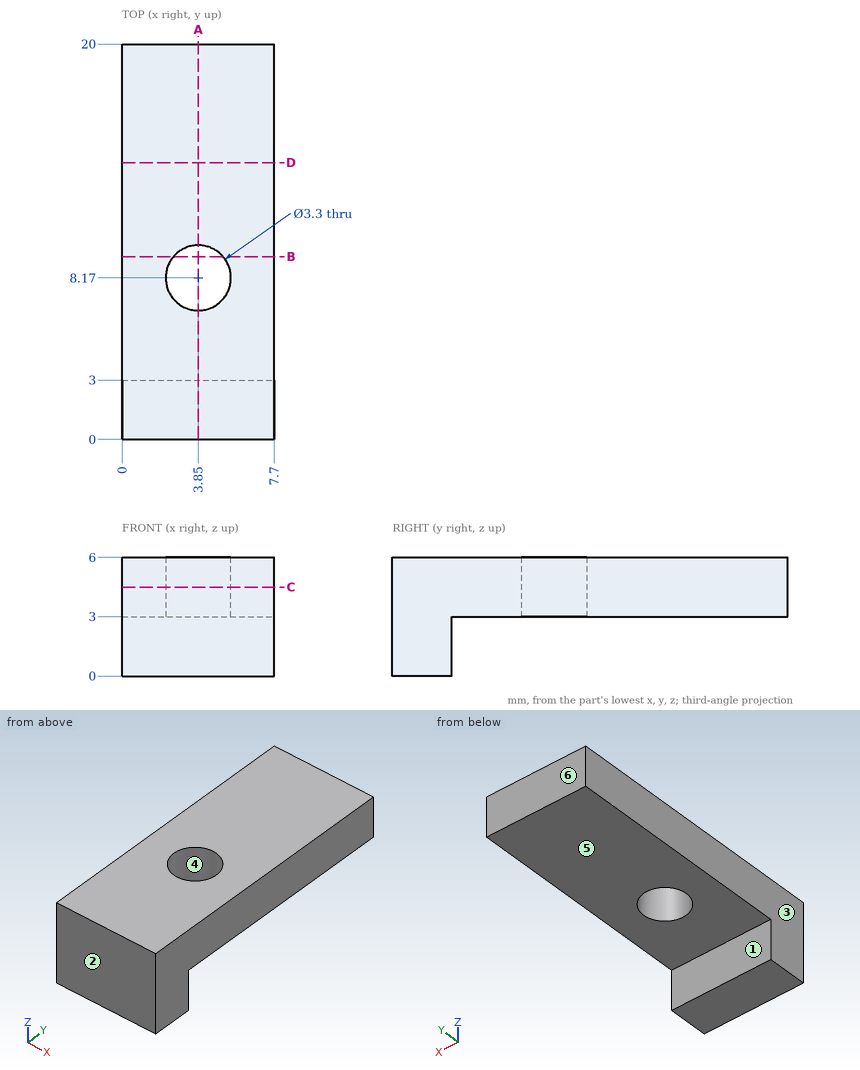
Study the drawing (mm; zero at the part's minimum x, y, z) and answer. A direction names the side the tool comes from. Coordinates: 2 decimals unless noted, no trailing zeros. Loops run counter-clockwise (first coordinate to the right, second up) from the corner with the lowest first, then second, coordinate; pieces in that order, holes last. Notation, with made-up numbers: M 56,83 L 111,83 A21 ccw 111,117 Z; hole C -32,-8.75 d2. An arc over 180 degrees is marked long. Answer in a Markdown table with one row per item. Add a question column.
1. Consider L1, parallel to Y at x = 3.85, z = 3.75; L2, parallel to Z at x = 0.5, y = 17.25; L3, parallel to Y at x = 1.5, z = 2.8. Determine where each line is inside the solid, lowest interval first.
2. The mould has two halves that part along Y. Classify the marked faces 1, 2, 3 and 4: pulls with the +Y half, pulls with the -Y half, needs draft (parallel to the pull), parting line crosses it, or undercut.
3. Find section B-B, the plane y = 9.25. Write down the section's boundary in (x, z).
4. A tool of negligible diameter and unlimited length cuts with its end or side. For the marked faces 5 and 6, from which of +Z, -Z, +X, -X, +Y, -Y can it reach the whole face along a straight path? Write none if from no direction.
5. Flat-ended cylindrical pins translate along their axes: P1, Ø4, axis at x = 5.5, y = 16, coming from the -Z side; P2, Ø2.5, axis at x = 2.5, z = 1.5, coming from the +Y side. Find the tip coordinate at first contact, or state that the pin passes through.
6. Find section D-D, the plane y = 14. Write down the section's boundary in (x, z).
7. Find section A-A, the plane x = 3.85. Write down the section's boundary in (y, z).
8. Find section C-C, the plane z = 4.5. Write down the section's boundary in (x, y).
Reported:
| question | item | result |
|---|---|---|
| 1 | L1 | y = 0 to 6.52, 9.82 to 20 |
| 1 | L2 | z = 3 to 6 |
| 1 | L3 | y = 0 to 3 |
| 2 | face 1 | pulls with the +Y half |
| 2 | face 2 | pulls with the -Y half |
| 2 | face 3 | needs draft |
| 2 | face 4 | undercut |
| 3 | outline | M 0,3 L 2.6,3 L 2.6,6 L 0,6 Z; M 5.1,3 L 7.7,3 L 7.7,6 L 5.1,6 Z |
| 4 | face 5 | -Z, +X, -X, +Y |
| 4 | face 6 | +Z, -Z, +X, -X, +Y |
| 5 | P1 | stops at z = 3 |
| 5 | P2 | stops at y = 3 |
| 6 | outline | M 0,3 L 7.7,3 L 7.7,6 L 0,6 Z |
| 7 | outline | M 0,0 L 3,0 L 3,3 L 6.52,3 L 6.52,6 L 0,6 Z; M 9.82,3 L 20,3 L 20,6 L 9.82,6 Z |
| 8 | outline | M 0,0 L 7.7,0 L 7.7,20 L 0,20 Z; hole C 3.85,8.17 d3.3 |
